from build123d import *

# Parameters (mm, degrees)
BOSS_EXTRUDE1_DEPTH = 9.45
SKETCH3_R           = 1.5
CUT_EXTRUDE1_DEPTH  = 3
SKETCH4_R           = 1.226272584
CUT_EXTRUDE2_DEPTH  = 3


with BuildPart() as part:
    # Sketch2 → Boss-Extrude1 (new, symmetric)
    with BuildSketch(Plane.XY):
        Polygon((-4.108578644, 6.75), (4.108578644, 6.75), (4.75, 6.108578644), (4.75, 5.101471863), (4.108578644, 4.460050506), (3.613603897, 4.460050506), (3.5, 4.346446609), (3.5, 3.753553391), (3.613603897, 3.639949494), (4.108578644, 3.639949494), (4.75, 2.998528137), (4.75, 2.257905525), (5.007905525, 2), (9.001471863, 2), (10, 2.998528137), (10, 9.001471863), (9.001471863, 10), (-9.001471863, 10), (-10, 9.001471863), (-10, 2.998528137), (-9.001471863, 2), (-5.007905525, 2), (-4.75, 2.257905525), (-4.75, 2.998528137), (-4.108578644, 3.639949494), (-3.613603897, 3.639949494), (-3.5, 3.753553391), (-3.5, 4.346446609), (-3.613603897, 4.460050506), (-4.108578644, 4.460050506), (-4.75, 5.101471863), (-4.75, 6.108578644), align=None)
    extrude(amount=BOSS_EXTRUDE1_DEPTH, both=True)

    # Sketch3 → Cut-Extrude1 (cut)
    with BuildSketch(Plane.XY.offset(9.45)):
        with Locations((-4.5, 8.25)):
            Circle(SKETCH3_R)
        with Locations(Location((4.5, 8.25, 0), (0, 0, 180))):
            Circle(SKETCH3_R)
    cut_extrude1 = extrude(amount=-CUT_EXTRUDE1_DEPTH, mode=Mode.SUBTRACT)

    # Mirror1: Cut-Extrude1 across plane
    add(cut_extrude1.mirror(Plane.XY), mode=Mode.SUBTRACT)

    # Sketch4 → Cut-Extrude2 (cut)
    with BuildSketch(Plane(origin=(0, 10, 0), x_dir=(1, 0, 0), z_dir=(0, 1, 0))):
        with Locations(Location((7.5, -5, 0), (0, 0, 270))):
            Circle(SKETCH4_R)
        with Locations(Location((-7.5, -5, 0), (0, 0, 90))):
            Circle(SKETCH4_R)
        with Locations(Location((-7.5, 5, 0), (0, 0, 270))):
            Circle(SKETCH4_R)
        with Locations(Location((7.5, 5, 0), (0, 0, 90))):
            Circle(SKETCH4_R)
    extrude(amount=-CUT_EXTRUDE2_DEPTH, mode=Mode.SUBTRACT)


solid = part.part
For this review, take the finished solid that the model builds, in its own axes (mm). A direction names the side the tool comes from. Give positions to 0.01 mm unless a question says otherwise; leave off trailing zeros. Loops run counter-clockwise (first coordinate to the right, second up) from the corner with the lowest first, then second, coordinate; pieces in that order, holes last.
Item 1: Tool access review of faces 1 (the cylindrical face through (-4.825, 6.786, 7.971)), 2 (the flat face through (7, 7, -5)), 3 (the flat face through (0, 6.75, 0)), 4 (the cylindrical face through (-4.825, 6.786, -7.971)), 5 (the flat face through (0, 7, 9.45)): name each direction out of +Z, -Z, +X, -X, +Y, -Y from which nothing blocks a thin tool from reaching the whole face with its end or side.
Item 2: Take a section at B-B, the plane y = 8.25. State the section outline as (x, z) points, and give its area (3 significant figures).
Item 3: Insertion check: pin 1 (1.8 mm diameter, centred on x = 4.5, y = 8.25, fed in from -Z); pin 2 (1.5 mm diameter, centred on x = -5, y = 8, fed in from +Z); pin 3 (6.5 mm diameter, centred on x = -0.5, z = 0, fed in from -Y). Each pin has a flat end and moves straight along its axis. Give the tip position at first contact, or say it passes through.
Item 4: Take a section at A-A, the plane y = 5.75. State the section outline as (x, z) points, and give its area (3 significant figures).
Item 5: For line 1 along X through (y, z) = (8.1, -5); line 2 along Y through (x, z) = (4.5, -8.6); line 3 along X through (y, z) = (8, 8.75), list the stretches that pass through material, from the lowest coordinate up.
Item 6: Take a section at D-D, the plane x = 7.5. State the section outline as (y, z) points.
Item 7: Take a section at C-C, the plane x = 4.5. State the section outline as (y, z) points.
Item 8: Draft analysis for pull direction Y (two halves, no side actions). For faces 6 (the flat face through (-4.75, 5.6, 0.1)), 7 (the cylindrical face through (4.825, 9.714, 7.971)), 8 (the cylindrical face through (8.697, 8.521, -4.734)), 9 (the flat face through (7, 2, 0)), state which applies: +Y half, -Y half, draft (parallel to the pull), parting line (faces both ways), or undercut.
Calculated:
1. face 1: +Z
1. face 2: +Y
1. face 3: +Z, -Z
1. face 4: -Z
1. face 5: +Z, +X, -X, +Y, -Y
2. outline: (-10, -9.45) - (-6, -9.45) - (-6, -6.45) - (-3, -6.45) - (-3, -9.45) - (3, -9.45) - (3, -6.45) - (6, -6.45) - (6, -9.45) - (10, -9.45) - (10, 9.45) - (6, 9.45) - (6, 6.45) - (3, 6.45) - (3, 9.45) - (-3, 9.45) - (-3, 6.45) - (-6, 6.45) - (-6, 9.45) - (-10, 9.45) - close; hole circle Ø2.45 at (-7.5, -5); hole circle Ø2.45 at (-7.5, 5); hole circle Ø2.45 at (7.5, -5); hole circle Ø2.45 at (7.5, 5)
2. area: 323 mm2
3. pin 1: stops at z = -6.45
3. pin 2: stops at z = 6.45
3. pin 3: stops at y = 3.64
4. outline: (-10, -9.45) - (-4.75, -9.45) - (-4.75, 9.45) - (-10, 9.45) - close; (4.75, -9.45) - (10, -9.45) - (10, 9.45) - (4.75, 9.45) - close
4. area: 198 mm2
5. line 1: x = -10 to -8.73, -6.27 to 6.27, 8.73 to 10
5. line 2: y = 3.25 to 4.85, 6.36 to 6.75, 9.75 to 10
5. line 3: x = -10 to -5.98, -3.02 to 3.02, 5.98 to 10
6. outline: (2, -9.45) - (10, -9.45) - (10, -6.23) - (7, -6.23) - (7, -3.77) - (10, -3.77) - (10, 3.77) - (7, 3.77) - (7, 6.23) - (10, 6.23) - (10, 9.45) - (2, 9.45) - close
7. outline: (3.25, -9.45) - (4.85, -9.45) - (4.85, 9.45) - (3.25, 9.45) - close; (6.36, -9.45) - (6.75, -9.45) - (6.75, -6.45) - (9.75, -6.45) - (9.75, -9.45) - (10, -9.45) - (10, 9.45) - (9.75, 9.45) - (9.75, 6.45) - (6.75, 6.45) - (6.75, 9.45) - (6.36, 9.45) - close
8. face 6: undercut
8. face 7: undercut
8. face 8: draft
8. face 9: -Y half
